Check sheet for the modelled part. Datum: model origin and axes. Units: mm. Face numbers are marked on the shaded views. A direction names the side the tool comes from. Coordinates: 2 decimals unless noted, no trailing zeros. Order: outer loops, then holes, each group sorted by start corner. A loop starts at its lowest first (then second) coordinate and runs counter-clockwise, first axis right, second up.
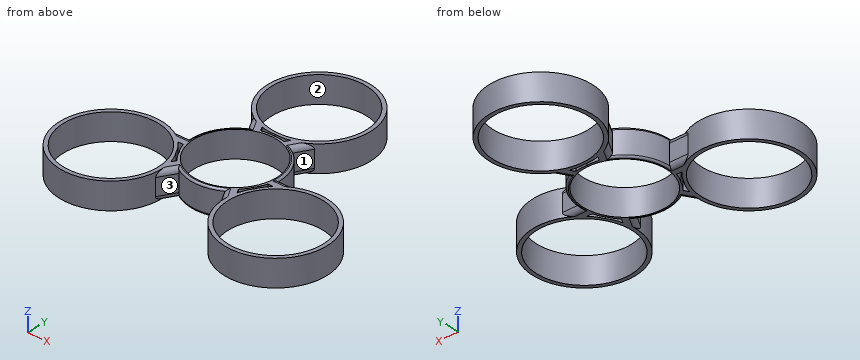
from build123d import *

# Parameters (mm, degrees)
F0_R     = 12.7
F0_R_2   = 11.1125
F1_DEPTH = 7.112
F2_R     = 1.27
F3_R     = 0.50799


# Not quite as in the source:
# - a fillet or chamfer is up to 0.001 mm smaller than in the source, because OpenCascade refuses the exact size
# - ends of sketch curves that miss each other by under 0.0002 mm in the source are joined


with BuildPart() as f1:
    # F0 (on Top) → F1 (new body)
    with BuildSketch(Plane.XY):
        with BuildLine():
            ThreePointArc((8.3638022209, 14.7734709329), (0, 39.3942033225), (-8.3638022209, 14.7734709329))
            Line((-8.3638022209, 14.7734709329), (-5.8662054787, 10.3931058657))
            ThreePointArc((-5.8662054787, 10.3931058657), (-10.3354618297, 5.9671806592), (-11.9337964262, -0.1162717145))
            Line((-11.9337964262, -0.1162717145), (-16.9761022194, -0.1434727603))
            ThreePointArc((-16.9761022194, -0.1434727603), (-34.1163779507, -19.6971066641), (-8.6122978741, -14.6300019249))
            Line((-8.6122978741, -14.6300019249), (-6.0675894575, -10.276836791))
            ThreePointArc((-6.0675894575, -10.276836791), (0, -11.934362834), (6.0675894575, -10.276836791))
            Line((6.0675894575, -10.276836791), (8.6122978741, -14.6300019249))
            ThreePointArc((8.6122978741, -14.6300019249), (34.1163779507, -19.6971066641), (16.9761022194, -0.1434727603))
            Line((16.9761022194, -0.1434727603), (11.9337964262, -0.1162717145))
            ThreePointArc((11.9337964262, -0.1162717145), (10.3354618297, 5.9671806592), (5.8662054787, 10.3931058657))
            Line((5.8662054787, 10.3931058657), (8.3638022209, 14.7734709329))
        make_face()
        with Locations((-22.225, -12.83160756)):
            Circle(F0_R, mode=Mode.SUBTRACT)
        with BuildLine():
            ThreePointArc((-8.9782080284, -9.6422017781), (-9.6052965229, -7.7965006784), (-10.5814479311, -6.109200777))
            ThreePointArc((-10.5814479311, -6.109200777), (-11.5546165578, -4.4201787661), (-12.8394961357, -2.9542534612))
            Line((-12.8394961357, -2.9542534612), (-11.4007424563, -2.9542534612))
            ThreePointArc((-11.4007424563, -2.9542534612), (-10.8372927454, -4.4313928826), (-10.042581953, -5.7980864121))
            ThreePointArc((-10.042581953, -5.7980864121), (-9.2563462346, -7.1696730271), (-8.258831006, -8.3962046475))
            Line((-8.258831006, -8.3962046475), (-8.9782080284, -9.6422017781))
        make_face(mode=Mode.SUBTRACT)
        with Locations((22.225, -12.83160756)):
            Circle(F0_R, mode=Mode.SUBTRACT)
        with BuildLine():
            Line((11.4007424563, -2.9542534612), (12.8394961357, -2.9542534612))
            ThreePointArc((12.8394961357, -2.9542534612), (11.5546165578, -4.4201787661), (10.5814479311, -6.109200777))
            ThreePointArc((10.5814479311, -6.109200777), (9.6052965229, -7.7965006784), (8.9782080284, -9.6422017781))
            Line((8.9782080284, -9.6422017781), (8.258831006, -8.3962046475))
            ThreePointArc((8.258831006, -8.3962046475), (9.2563462346, -7.1696730271), (10.042581953, -5.7980864121))
            ThreePointArc((10.042581953, -5.7980864121), (10.8372927454, -4.4313928826), (11.4007424563, -2.9542534612))
        make_face(mode=Mode.SUBTRACT)
        Circle(F0_R_2, mode=Mode.SUBTRACT)
        with BuildLine():
            ThreePointArc((-3.8612913684, 12.5964559897), (-1.9493229697, 12.2166805672), (-2.6876e-06, 12.2184031057))
            ThreePointArc((-2.6876e-06, 12.2184031057), (1.9493202828, 12.2166814247), (3.8612885145, 12.5964576884))
            Line((3.8612885145, 12.5964576884), (3.1419093526, 11.3504602412))
            ThreePointArc((3.1419093526, 11.3504602412), (1.5809467105, 11.6010677307), (0, 11.5961742969))
            ThreePointArc((0, 11.5961742969), (-1.5809492634, 11.6010670352), (-3.141914346, 11.350458859))
            Line((-3.141914346, 11.350458859), (-3.8612913684, 12.5964559897))
        make_face(mode=Mode.SUBTRACT)
        with Locations((0, 25.6632216382)):
            Circle(F0_R, mode=Mode.SUBTRACT)
    extrude(amount=F1_DEPTH)

    # F2
    f2_edges = [f1.edges().sort_by_distance(p)[0] for p in [
        (-7.339944, -12.453419, 7.112),
        (-14.454949, -0.129872, 7.112),
        (7.339944, -12.453419, 7.112),
        (14.454949, -0.129872, 7.112),
        (7.115004, 12.583288, 7.112),
        (-7.115004, 12.583288, 7.112),
        (-7.339944, -12.453419, 0),
        (7.339944, -12.453419, 0),
        (14.454949, -0.129872, 0),
        (7.115004, 12.583288, 0),
        (-7.115004, 12.583288, 0),
        (-14.454949, -0.129872, 0),
    ]]
    fillet(f2_edges, radius=F2_R)

    # F3 (radius 0.508 in the source; OpenCascade refuses exactly that, so slightly less here)
    f3_edges = [f1.edges().sort_by_distance(p)[0] for p in [
        (-10.335462, 5.967181, 7.112),
        (0, -11.934363, 7.112),
        (10.335462, 5.967181, 7.112),
        (10.335462, 5.967181, 0),
        (-10.335462, 5.967181, 0),
        (0, -11.934363, 0),
    ]]
    fillet(f3_edges, radius=F3_R)


solid = f1.part
(1) Cross-section at B-B (y = 21.5). Enter the section's corners in (x, z), and give its area (3 significant figures).
Filled in:
outline: (-13.08, 0) - (-12, 0) - (-12, 7.11) - (-13.08, 7.11) - close; (12, 0) - (13.08, 0) - (13.08, 7.11) - (12, 7.11) - close
area: 15.5 mm2
(2) Cross-section at C-C (z = 5). Count the separate pieces of the cut face and the enclosed holes in it, and give its area (3 significant figures).
Filled in:
separate pieces: 1
enclosed holes: 7
area: 355 mm2
(3) Go/stop test with flat-tipped pins: P1, Ø23, axis at x = -22.22, y = -12.83, coming from the +Z side; P2, Ø4, axis at y = 18, z = 2.5, coming from the +X side; P3, Ø10, axis at x = -13, y = -14.5, coming from the +Z side; P4, Ø3, axis at y = -8, z = 3, coming from the +X side. Record where each tip stops, or that it passes through.
Filled in:
P1: passes through
P2: stops at x = 12.51
P3: stops at z = 7.11
P4: stops at x = 35.55
(4) Cross-section at A-A (x = 29). Enter the section's corners in (y, z), and give its area (3 significant figures).
Filled in:
outline: (-24.77, 0) - (-23.57, 0) - (-23.57, 7.11) - (-24.77, 7.11) - close; (-2.09, 0) - (-0.89, 0) - (-0.89, 7.11) - (-2.09, 7.11) - close
area: 17.1 mm2
(5) Tool access check on the marked faces 1, 2 and 3. Record the directions out of +Z, -Z, +X, -X, +Y, -Y that give a thin tool (end or side, any length) a straight path to the whole face; none if there is none.
Filled in:
face 1: +Z, -Z, +X
face 2: +Z, -Z
face 3: +Z, -Z, -Y
(6) Thickness scan on probe 1 along Y at (x, z) = (0, 5.75); probe 2 along X at (y, z) = (-22.5, 6.25); probe 3 along Y at (x, z) = (-8, 5.5). Record the ranges inside material, lowest first.
Filled in:
probe 1: y = -11.93 to -11.11, 11.11 to 11.6, 12.22 to 12.96, 38.36 to 39.39
probe 2: x = -31.97 to -30.46, -13.99 to -12.48, 12.48 to 13.99, 30.46 to 31.97
probe 3: y = -13.58 to -7.71, 7.71 to 8.86, 14.14 to 15.8, 35.53 to 36.82
